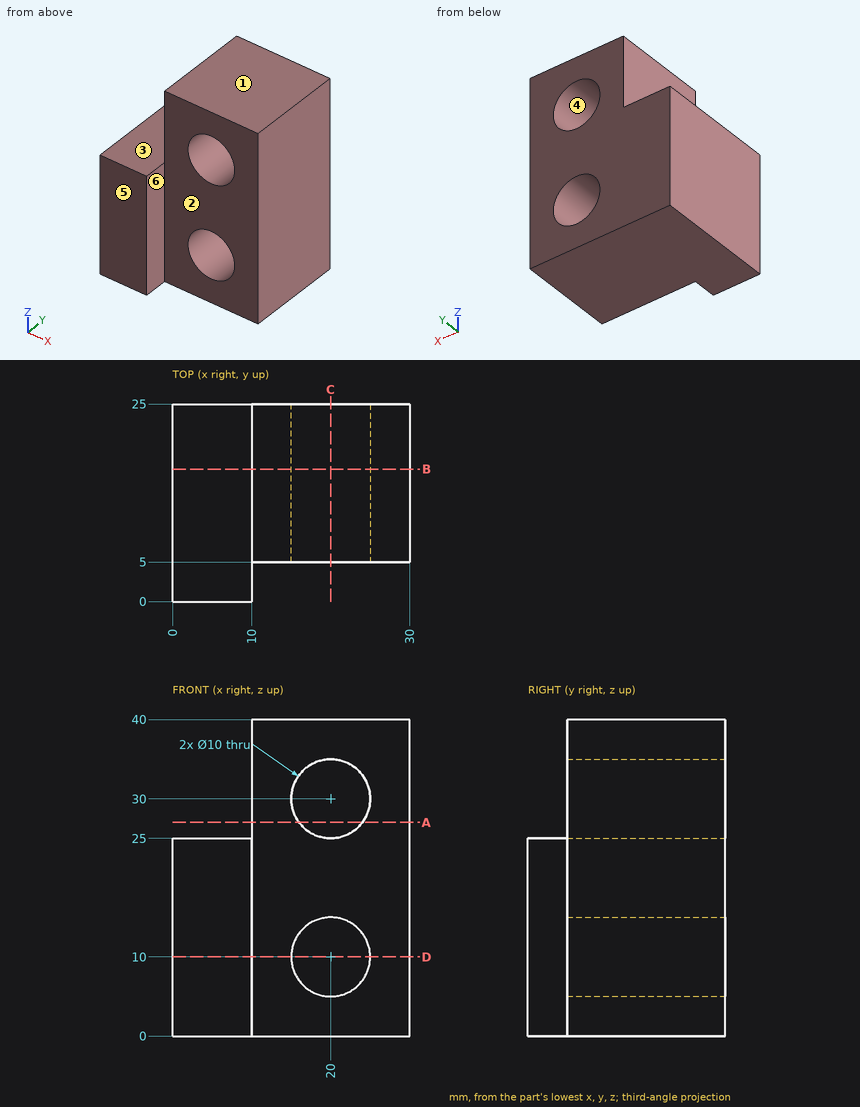
Design review of the part shown in the three views and the two pictorial views. Dimensions are in mm from the part's minimum x, y and z. A direction names the side the tool comes from. Round coordinates to 2 decimals unless told otherwise and drop trailing zeros. Loops run counter-clockwise (first coordinate to the right, second up) from the corner with the lowest first, then second, coordinate; pieces in that order, holes last. Notation, with made-up numbers: (-22.5, -3) -> (3.5, -3) arc R10 cw to (3.5, 10) -> close; hole circle Ø2 at (65.25, 64). An arc over 180 degrees is marked (long way). Answer as CSV lines item,"result".
1) Add section C-C on x = 20. Write out the cut boundary in (y, z), plus the area to 3 significant figures.
Geometry results:
outline,"(5, 0) -> (25, 0) -> (25, 5) -> (5, 5) -> close; (5, 15) -> (25, 15) -> (25, 25) -> (5, 25) -> close; (5, 35) -> (25, 35) -> (25, 40) -> (5, 40) -> close"
area,"400 mm²"
2) Add section B-B on y = 16.75. Write out the cut boundary in (x, z).
Geometry results:
outline,"(0, 0) -> (30, 0) -> (30, 40) -> (10, 40) -> (10, 25) -> (0, 25) -> close; hole circle Ø10 at (20, 10); hole circle Ø10 at (20, 30)"
3) For P1, Ø7.5, axis at y = 12, z = 32.5, coming from the -X side; P2, Ø12, axis at x = 6.5, y = 15, coming from the +Z side; P3, Ø5, axis at x = 5.5, y = 12.5, coming from the +Z side; P4, Ø6, axis at x = 22, z = 16.5, coming from the -Y side, all flat-tipped, find the tip position at first contact; note any pin that passes through.
Geometry results:
P1,"stops at x = 10"
P2,"stops at z = 40"
P3,"stops at z = 25"
P4,"stops at y = 5"
4) Add section A-A on z = 27. Write out the cut boundary in (x, y), plus the area to 3 significant figures.
Geometry results:
outline,"(10, 5) -> (16, 5) -> (16, 25) -> (10, 25) -> close; (24, 5) -> (30, 5) -> (30, 25) -> (24, 25) -> close"
area,"240 mm²"
5) Tool access review of the marked faces 1, 2 and 3: name each direction out of +Z, -Z, +X, -X, +Y, -Y from which nothing blocks a thin tool from reaching the whole face with its end or side.
Geometry results:
face 1,"+Z, +X, -X, +Y, -Y"
face 2,"+Z, -Z, +X, -Y"
face 3,"+Z, -X, +Y, -Y"
6) Draft analysis for pull direction X (two halves, no side actions). For the marked faces 4, 5 and 6, state which applies: pulls with the +X half, pulls with the -X half, needs draft (parallel to the pull), parting line crosses it, or undercut.
Geometry results:
face 4,"undercut"
face 5,"needs draft"
face 6,"pulls with the +X half"
7) Add section D-D on z = 10. Write out the cut boundary in (x, y).
Geometry results:
outline,"(0, 0) -> (10, 0) -> (10, 5) -> (15, 5) -> (15, 25) -> (0, 25) -> close; (25, 5) -> (30, 5) -> (30, 25) -> (25, 25) -> close"
8) To check wall thickness, follow line 1 along Z through (x, y) = (20, 20.5); line 2 along Z through (x, y) = (24.5, 20.5); line 3 along X through (y, z) = (15, 30). State the ranges of each line that lie inside material, in increasing order. Write a range as from..to.
Geometry results:
line 1,"z = 0..5, 15..25, 35..40"
line 2,"z = 0..7.82, 12.18..27.82, 32.18..40"
line 3,"x = 10..15, 25..30"
